The model under review builds one solid part; all positions refer to its coordinate system, in mm. A direction names the side the tool comes from. Round coordinates to 2 decimals unless told otherwise and drop trailing zeros. Write each loop counter-clockwise with the first axis right and the second up, starting at its lowest first coordinate (ties: lowest second). Pieces come first, ordered by that corner, then holes. Notation, with made-up numbers: M 88,-6 L 134,-6 A19 ccw 134,19 Z; hole C -10,56.5 d7. An arc over 180 degrees is marked long. One line per item, written item: value. Start each with the question number.
1) Take a section at A-A, the plane z = 6.5. Write out the cut boundary in (x, y).
2) Tool access review of faces 5 (the face through (5.259, 10, 13)), 6 (the face through (5.881, -9.033, 10.278)), 7 (the face through (7.27, -4.12, 4.16)): name each direction out of +Z, -Z, +X, -X, +Y, -Y from which nothing blocks a thin tool from reaching the whole face with its end or side.
3) Take a section at B-B, the plane z = 12.25. State how many separate pieces and enclosed holes the cut face has, and give its area (3 significant figures).
4) For P1, Ø8, axis at x = -3.5, y = 7, coming from the +Z side; P2, Ø12, axis at x = 7.5, z = 14.5, coming from the -Y side; P3, Ø3, axis at y = 7, z = 2, coming from the -X side, all flat-tipped, find the tip position at first contact; note any pin that passes through.
5) Mouldability with a two-part tool opening along X and no side actions: class faces 1 (the face through (0.08, -11.39, 8.71)), 2 (the face through (-10, 6, 17.667)), 3 (the face through (-0.115, -13.928, 7.079)), 4 (the face through (-9.47, -5.39, 3.78)) as +X half, -X half, draft (parallel to the pull), parting line (faces both ways), or undercut.
6) Take a section at D-D, the plane z = -1.25. Write out the cut boundary in (x, y), and give its area (3 significant figures).
7) Wall thickness on probe 1 along Y at (x, z) = (0, 5); probe 2 along Z at (x, y) = (-8.5, 0.5); probe 3 along X at (y, z) = (-2.25, 9.75): over which ranges is each line inside the solid? List them lowest first.
8) Take a section at C-C, the plane y = 6.5. Write out the cut boundary in (x, z), and give its area (3 significant figures).
from build123d import *

# Parameters (mm, degrees)
F2_DEPTH  = 17.6665466667
F3_DEPTH  = 3.81
F5_W      = 10.4865888134
F5_H      = 7.7739614062
F6_DEPTH  = 30.1752
F8_W      = 10.48512
F8_H      = 7.7724
F9_DEPTH  = 32.004
F11_W     = 10.48512
F11_H     = 7.7724
F12_DEPTH = 31.6738
F13_R     = 2.54
F14_R     = 1.27


with BuildPart() as f2:
    # F1 (on Top) → F2 (new body)
    with BuildSketch(Plane.XY):
        with BuildLine():
            Line((6.8124849158, -9.9955756726), (12.0626649158, -0.9019971637))
            ThreePointArc((12.0626649158, -0.9019971637), (12.0626649158, 6.9643828363), (5.25018, 10.8975728363))
            Line((5.25018, 10.8975728363), (-5.25018, 10.8975728363))
            ThreePointArc((-5.25018, 10.8975728363), (-12.0626649158, 6.9643828363), (-12.0626649158, -0.9019971637))
            Line((-12.0626649158, -0.9019971637), (-6.8124849158, -9.9955756726))
            ThreePointArc((-6.8124849158, -9.9955756726), (0, -13.9287656726), (6.8124849158, -9.9955756726))
        make_face()
        with BuildLine():
            ThreePointArc((-9.8629603902, 0.3680028363), (-9.8629603902, 5.6943828363), (-5.25018, 8.3575728363))
            Line((-5.25018, 8.3575728363), (5.25018, 8.3575728363))
            ThreePointArc((5.25018, 8.3575728363), (9.8629603902, 5.6943828363), (9.8629603902, 0.3680028363))
            Line((9.8629603902, 0.3680028363), (4.6127803902, -8.7255756726))
            ThreePointArc((4.6127803902, -8.7255756726), (0, -11.3887656726), (-4.6127803902, -8.7255756726))
            Line((-4.6127803902, -8.7255756726), (-9.8629603902, 0.3680028363))
        make_face(mode=Mode.SUBTRACT)
    extrude(amount=F2_DEPTH)

    # F1 (on Top) → F3 (join)
    with BuildSketch(Plane.XY):
        with BuildLine():
            Line((6.8124849158, -9.9955756726), (12.0626649158, -0.9019971637))
            ThreePointArc((12.0626649158, -0.9019971637), (12.0626649158, 6.9643828363), (5.25018, 10.8975728363))
            Line((5.25018, 10.8975728363), (-5.25018, 10.8975728363))
            ThreePointArc((-5.25018, 10.8975728363), (-12.0626649158, 6.9643828363), (-12.0626649158, -0.9019971637))
            Line((-12.0626649158, -0.9019971637), (-6.8124849158, -9.9955756726))
            ThreePointArc((-6.8124849158, -9.9955756726), (0, -13.9287656726), (6.8124849158, -9.9955756726))
        make_face()
        with BuildLine():
            ThreePointArc((-9.8629603902, 0.3680028363), (-9.8629603902, 5.6943828363), (-5.25018, 8.3575728363))
            Line((-5.25018, 8.3575728363), (5.25018, 8.3575728363))
            ThreePointArc((5.25018, 8.3575728363), (9.8629603902, 5.6943828363), (9.8629603902, 0.3680028363))
            Line((9.8629603902, 0.3680028363), (4.6127803902, -8.7255756726))
            ThreePointArc((4.6127803902, -8.7255756726), (0, -11.3887656726), (-4.6127803902, -8.7255756726))
            Line((-4.6127803902, -8.7255756726), (-9.8629603902, 0.3680028363))
        make_face(mode=Mode.SUBTRACT)
        with BuildLine():
            Line((5.25018, 8.3575728363), (-5.25018, 8.3575728363))
            ThreePointArc((-5.25018, 8.3575728363), (-9.8629603902, 5.6943828363), (-9.8629603902, 0.3680028363))
            Line((-9.8629603902, 0.3680028363), (-4.6127803902, -8.7255756726))
            ThreePointArc((-4.6127803902, -8.7255756726), (0, -11.3887656726), (4.6127803902, -8.7255756726))
            Line((4.6127803902, -8.7255756726), (9.8629603902, 0.3680028363))
            ThreePointArc((9.8629603902, 0.3680028363), (9.8629603902, 5.6943828363), (5.25018, 8.3575728363))
        make_face()
    extrude(amount=-F3_DEPTH)

    # F5 (on offset) → F6 (cut)
    with BuildSketch(Plane(origin=(-31.4346201719, -18.1487864181, 0), x_dir=(0.5, -0.8660254038, 0), z_dir=(-0.8660254038, -0.5, 0))):
        with Locations((0.0030086376, 14.4617783371)):
            Rectangle(F5_W, F5_H)
    extrude(amount=-F6_DEPTH, mode=Mode.SUBTRACT)

    # F8 (on offset) → F9 (cut)
    with BuildSketch(Plane(origin=(0, 36.2975728363, 0), x_dir=(-1, 0, 0), z_dir=(0, 1, 0))):
        with Locations((-0.0165903475, 13.8303037011)):
            Rectangle(F8_W, F8_H)
    extrude(amount=-F9_DEPTH, mode=Mode.SUBTRACT)

    # F11 (on offset) → F12 (cut)
    with BuildSketch(Plane(origin=(31.4346201719, -18.1487864181, 0), x_dir=(0.5, 0.8660254038, 0), z_dir=(0.8660254038, -0.5, 0))):
        with Locations((-0.0020326115, 13.782461328)):
            Rectangle(F11_W, F11_H)
    extrude(amount=-F12_DEPTH, mode=Mode.SUBTRACT)

    # F13
    f13_edges = [f2.edges().sort_by_distance(p)[0] for p in [
        (5.25915, 9.627567, 17.666547),
        (-5.22597, 9.627573, 17.666547),
        (5.715426, -9.355737, 17.666547),
        (10.957986, -0.275357, 17.666547),
        (-5.714571, -9.357218, 17.666547),
        (-10.957866, -0.275566, 17.666547),
    ]]
    fillet(f13_edges, radius=F13_R)

    # F14
    f14_edges = [f2.edges().sort_by_distance(p)[0] for p in [
        (-5.714571, -9.357218, 10.574798),
        (5.25915, 9.627567, 9.944104),
        (-5.22597, 9.627573, 9.944104),
        (5.715426, -9.355737, 9.896261),
        (10.957986, -0.275357, 9.896261),
        (-10.957866, -0.275566, 10.574798),
    ]]
    fillet(f14_edges, radius=F14_R)


solid = f2.part
Checked values:
1. outline: M -12.06,-0.9 L -6.81,-10 A7.87 ccw 6.81,-10 L 12.06,-0.9 A7.87 ccw 5.25,10.9 L -5.25,10.9 A7.87 ccw Z; hole M -9.86,0.37 L -4.61,-8.73 A5.33 ccw 4.61,-8.73 L 9.86,0.37 A5.33 ccw 5.25,8.36 L -5.25,8.36 A5.33 ccw Z
2. face 5: +Z, +Y
2. face 6: +Z, +X
2. face 7: +Z
3. separate pieces: 3
3. enclosed holes: 0
3. area: 105 mm2
4. P1: stops at z = 17.64
4. P2: stops at y = -13.78
4. P3: stops at x = -12.72
5. face 1: undercut
5. face 2: draft
5. face 3: parting line
5. face 4: -X half
6. outline: M -12.06,-0.9 L -6.81,-10 A7.87 ccw 6.81,-10 L 12.06,-0.9 A7.87 ccw 5.25,10.9 L -5.25,10.9 A7.87 ccw Z
6. area: 490 mm2
7. probe 1: y = -13.93 to -11.39, 8.36 to 10.9
7. probe 2: z = -3.81 to 0
7. probe 3: x = -11.28 to -8.35, 8.35 to 11.28
8. outline: M -12.31,-3.81 L 12.31,-3.81 L 12.31,17.67 L 9.29,17.67 L 9.29,0 L -9.29,0 L -9.29,17.67 L -12.31,17.67 Z
8. area: 200 mm2
